Work out the finished part from the listing and answer in its coordinate system (mm). Face numbers are marked on the shaded views. Round coordinates to 2 decimals unless told otherwise and drop trailing zeros. Write each loop counter-clockwise with the first axis right and the second up, starting at its lowest first coordinate (ties: lowest second). Pieces come first, ordered by that corner, then holes. Notation, with made-up numbers: (0, 35) -> (45, 35) arc R15 cw to (45, 60) -> close; hole circle Ø9 at (34, 59.5). An arc over 180 degrees is marked (long way). One line per item, written item: value.
Autodesk Inventor part; units mm, degrees
ref_plane "YZ Plane" through (0, 0, 0) normal (1, 0, 0) x (0, 1, 0)
ref_plane "XZ Plane" through (0, 0, 0) normal (0, 1, 0) x (-1, 0, 0)
ref_plane "XY Plane" through (0, 0, 0) normal (0, 0, 1) x (1, 0, 0)
sketch "Sketch1" plane through (0, 0, 0) normal (0, 1, 0) x (-1, 0, 0)
  circle A0 centre (9, 0) radius 1.9
  circle A1 centre (4.5, 7.7942) radius 1.9
  circle A2 centre (-4.5, 7.7942) radius 1.9
  circle A3 centre (-9, 0) radius 1.9
  circle A4 centre (-4.5, -7.7942) radius 1.9
  circle A5 centre (4.5, -7.7942) radius 1.9
  circle A6 centre (9, 0) radius 4.3
  circle A7 centre (4.5, 7.7942) radius 4.3
  circle A8 centre (-4.5, 7.7942) radius 4.3
  circle A9 centre (-9, 0) radius 4.3
  circle A10 centre (-4.5, -7.7942) radius 4.3
  circle A11 centre (4.5, -7.7942) radius 4.3
  circle A12 centre (0, 0) radius 10.9
  circle A13 centre (0, 0) radius 2.25
  circle A14 centre (0, 0) radius 4.7
  dimension "d0" = 3.8
  dimension "d1" = 9
  dimension "d4" = 360
  dimension "d6" = 2.4
  dimension "d9" = 360
  dimension "d13" = 4.5
  dimension "d30" = 8.6
extrude "Extrusion1" add sketch "Sketch1" along normal mid plane 13 contours A12 A6 | A12 A6 | A6 A14 A7 A12 | A12 A11 A14 A6 | A14 | A12 A7 | A7 A12 | A12 A11 | A11 A12 | A14 A8 A12 A7 | A11 A12 A10 A14 | A14 A9 A12 A8 | A8 A12 | A10 A12 | A10 A12 A9 A14 | A12 A8 | A9 A12 | A10 A12 | A12 A9 | A13
extrude "Extrusion2" cut sketch "Sketch1" along normal through all both and the other way through all contours A13
extrude "Extrusion3" cut sketch "Sketch1" along normal mid plane 5 contours A0 | A12 A6 | A12 A6 | A6 A14 A7 A12 | A12 A11 A14 A6 | A14 | A12 A7 | A1 | A7 A12 | A5 | A12 A11 | A11 A12 | A14 A8 A12 A7 | A11 A12 A10 A14 | A14 A9 A12 A8 | A2 | A8 A12 | A4 | A10 A12 | A10 A12 A9 A14 | A12 A8 | A3 | A9 A12 | A10 A12 | A12 A9
extrude "Extrusion4" add sketch "Sketch1" along normal through all both and the other way through all contours A14
hole "Hole1" at (0, 6.5, 0) direction (0, -1, 0) diameter 5 end through all counterbore diameter 8 counterbore depth 2
mirror "Mirror1" about plane through (0, 0, 0) normal (0, 1, 0) of "Hole1"
properties part number "piston-star-connector"
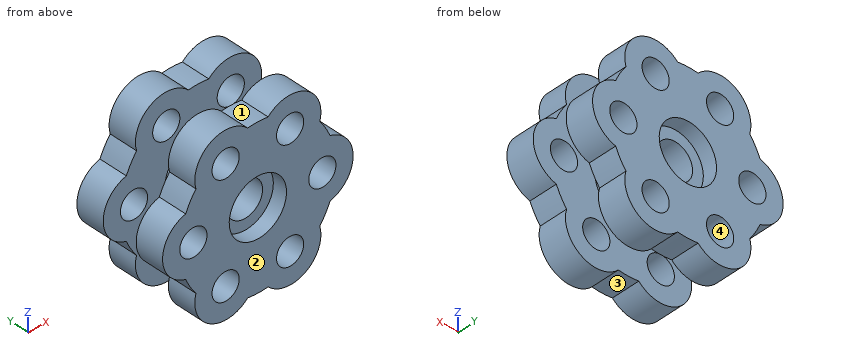
(1) Consider probe 1 along Z at (x, y) = (-4.5, -3.95); probe 2 along X at (y, z) = (-5.5, 9); probe 3 along Y at (x, z) = (0.25, 8). Determine where each line is inside the solid, lowest interval first.
Reported:
probe 1: z = -12.09 to -9.69, -5.89 to 5.89, 9.69 to 12.09
probe 2: x = -8.63 to -5.97, -3.03 to 3.03, 5.97 to 8.63
probe 3: y = -6.5 to -2.5, 2.5 to 6.5
(2) Find section C-C on y = -4. Give the vertices of the cut face in (x, z), plus the area to 3 significant figures.
Reported:
outline: (-10.07, -4.16) arc R10.9 ccw to (-8.64, -6.64) arc R4.3 ccw to (-1.43, -10.81) arc R10.9 ccw to (1.43, -10.81) arc R4.3 ccw to (8.64, -6.64) arc R10.9 ccw to (10.07, -4.16) arc R4.3 ccw to (10.07, 4.16) arc R10.9 ccw to (8.64, 6.64) arc R4.3 ccw to (1.43, 10.81) arc R10.9 ccw to (-1.43, 10.81) arc R4.3 ccw to (-8.64, 6.64) arc R10.9 ccw to (-10.07, 4.16) arc R4.3 ccw to start; hole circle Ø3.8 at (-9, 0); hole circle Ø3.8 at (-4.5, -7.79); hole circle Ø3.8 at (-4.5, 7.79); hole circle Ø5 at (0, 0); hole circle Ø3.8 at (4.5, -7.79); hole circle Ø3.8 at (4.5, 7.79); hole circle Ø3.8 at (9, 0)
area: 377 mm2
(3) Find section B-B on z = 5.5. Give the vertices of the cut face in (x, y).
Reported:
outline: (-9.41, -6.5) -> (9.41, -6.5) -> (9.41, -2.5) -> (-9.41, -2.5) -> close; (-9.41, 2.5) -> (9.41, 2.5) -> (9.41, 6.5) -> (-9.41, 6.5) -> close
(4) Find section D-D on z = -6.25. Give the vertices of the cut face in (x, y), plus the area to 3 significant figures.
Reported:
outline: (-8.93, -6.5) -> (-5.61, -6.5) -> (-5.61, -2.5) -> (-8.93, -2.5) -> close; (-8.93, 2.5) -> (-5.61, 2.5) -> (-5.61, 6.5) -> (-8.93, 6.5) -> close; (-3.39, -6.5) -> (3.39, -6.5) -> (3.39, -2.5) -> (-3.39, -2.5) -> close; (-3.39, 2.5) -> (3.39, 2.5) -> (3.39, 6.5) -> (-3.39, 6.5) -> close; (5.61, -6.5) -> (8.93, -6.5) -> (8.93, -2.5) -> (5.61, -2.5) -> close; (5.61, 2.5) -> (8.93, 2.5) -> (8.93, 6.5) -> (5.61, 6.5) -> close
area: 107 mm2
(5) Flat-ended cylindrical pins translate along their axes: pin 1 Ø4 at (x, z) = (-1.5, 1) entering from -Y; pin 2 Ø5 at (y, z) = (-4.5, -8.5) entering from -X. Find the tip coordinate at first contact, or state that the pin passes through.
Reported:
pin 1: stops at y = -4.5
pin 2: stops at x = -9.1
(6) For a pull along Z with two mould halves and no side action, classify the marked faces 1, 2, 3 and 4 as pulls with the +Z half, pulls with the -Z half, needs draft (parallel to the pull), parting line crosses it, or undercut.
Reported:
face 1: pulls with the +Z half
face 2: needs draft
face 3: pulls with the -Z half
face 4: undercut
(7) Find section A-A on x = 0. Give the vertices of the cut face in (y, z), plus the area to 3 significant figures.
Reported:
outline: (-6.5, -10.9) -> (-2.5, -10.9) -> (-2.5, -4.7) -> (2.5, -4.7) -> (2.5, -10.9) -> (6.5, -10.9) -> (6.5, -4) -> (4.5, -4) -> (4.5, -2.5) -> (-4.5, -2.5) -> (-4.5, -4) -> (-6.5, -4) -> close; (-6.5, 4) -> (-4.5, 4) -> (-4.5, 2.5) -> (4.5, 2.5) -> (4.5, 4) -> (6.5, 4) -> (6.5, 10.9) -> (2.5, 10.9) -> (2.5, 4.7) -> (-2.5, 4.7) -> (-2.5, 10.9) -> (-6.5, 10.9) -> close
area: 144 mm2
